Model file for the job. Use its own axes, mm. A direction names the side the tool comes from. Give positions to 0.01 mm unless a question says otherwise; leave off trailing zeros. Loops run counter-clockwise (first coordinate to the right, second up) from the corner with the lowest first, then second, coordinate; pieces in that order, holes last. Notation, with made-up numbers: (-34, 50) - (12, 50) arc R25 cw to (12, 80) - close; hole circle Ø6 at (12.25, 3). An arc over 180 degrees is marked (long way). Use a Markdown table: item, result.
from build123d import *

# Parameters (mm, degrees)
F0_W          = 12.7
F0_H          = 12.7
F1_DEPTH      = 16.51
F1_DEPTH_BACK = 16.51
F2_W          = 27.94
F2_H          = 6.35
F3_DEPTH      = 25.4
F5_DEPTH      = 27.94
F7_D          = 3.81
F8_R          = 3.81
F9_DEPTH      = 1.27


with BuildPart() as f1:
    # F0 (on Right) → F1 (new body, two sides)
    with BuildSketch(Plane.YZ) as f1_sk:
        Rectangle(F0_W, F0_H)
    extrude(amount=F1_DEPTH)
    extrude(f1_sk.sketch, amount=-F1_DEPTH_BACK)

    # F2 (on face) → F3 (cut)
    with BuildSketch(Plane.XZ.offset(6.35)):
        with Locations((0, -3.175)):
            Rectangle(F2_W, F2_H)
    extrude(amount=-F3_DEPTH, mode=Mode.SUBTRACT)

    # F4 (on face) → F5 (cut)
    with BuildSketch(Plane(origin=(13.97, 0, 0), x_dir=(0, -1, 0), z_dir=(-1, 0, 0))):
        with BuildLine():
            Line((-6.35, 0), (6.35, 0))
            ThreePointArc((6.35, 0), (0, 2.430635), (-6.35, 0))
        make_face()
    extrude(amount=F5_DEPTH, mode=Mode.SUBTRACT)

    # F7 (through all)
    with Locations(Plane.YZ.offset(16.51)):
        with Locations((0, -0.762)):
            Hole(F7_D / 2)

    # F8 (on face) → F9 (join)
    with BuildSketch(Plane.XY.offset(6.35)):
        with Locations((-10.16, 0)):
            Circle(F8_R)
        Circle(F8_R)
        with Locations((10.16, 0)):
            Circle(F8_R)
    extrude(amount=F9_DEPTH)


solid = f1.part
(1) Slice it at A-A, the plane z = -4.5. Write the cut outline in (x, y).
Computed:
| item | result |
|---|---|
| outline | (-16.51, -6.35) - (-13.97, -6.35) - (-13.97, 6.35) - (-16.51, 6.35) - close; (13.97, -6.35) - (16.51, -6.35) - (16.51, 6.35) - (13.97, 6.35) - close |
(2) Mould opens along Y. For faces 1 (the cylindrical face through (0.2, -0.1, 2.43)), 2 (the cylindrical face through (15.222, -1.817, -0.19)), 3 (the flat face through (0, 6.35, 3)), 4 (the cylindrical face through (6.354, 0.168, 6.976)) say: pulls with the +Y half, pulls with the -Y half, needs draft (parallel to the pull), parting line crosses it, or undercut.
Computed:
| item | result |
|---|---|
| face 1 | undercut |
| face 2 | undercut |
| face 3 | pulls with the +Y half |
| face 4 | parting line crosses it |
(3) Pin check, flat tips, straight feed: P1, Ø6, axis at y = 0, z = -0.762, coming from the +X side; P2, Ø3.5, axis at y = 0, z = -0.762, coming from the +X side; P3, Ø6, axis at x = 0, y = -2.5, coming from the -Z side. Stop position of each tip, or through.
Computed:
| item | result |
|---|---|
| P1 | x = 16.51 |
| P2 | through |
| P3 | z = 0.68 |
(4) Slice it at D-D, the plane y = -3. Write the cut outline in (x, z).
Computed:
| item | result |
|---|---|
| outline | (-16.51, -6.35) - (-13.97, -6.35) - (-13.97, 1.95) - (13.97, 1.95) - (13.97, -6.35) - (16.51, -6.35) - (16.51, 6.35) - (12.51, 6.35) - (12.51, 7.62) - (7.81, 7.62) - (7.81, 6.35) - (2.35, 6.35) - (2.35, 7.62) - (-2.35, 7.62) - (-2.35, 6.35) - (-7.81, 6.35) - (-7.81, 7.62) - (-12.51, 7.62) - (-12.51, 6.35) - (-16.51, 6.35) - close |
(5) Slice it at C-C, the plane x = 10.16. Write the cut outline in (y, z), plus the area to 3 significant figures.
Computed:
| item | result |
|---|---|
| outline | (-6.35, 0) arc R9.51 cw to (6.35, 0) - (6.35, 6.35) - (3.81, 6.35) - (3.81, 7.62) - (-3.81, 7.62) - (-3.81, 6.35) - (-6.35, 6.35) - close |
| area | 69.2 mm² |
(6) Slice it at B-B, the plane y = 0. Write the cut outline in (x, z), plus the area to 3 significant figures.
Computed:
| item | result |
|---|---|
| outline | (-16.51, -6.35) - (-13.97, -6.35) - (-13.97, -2.67) - (-16.51, -2.67) - close; (-16.51, 1.14) - (-13.97, 1.14) - (-13.97, 2.43) - (13.97, 2.43) - (13.97, 1.14) - (16.51, 1.14) - (16.51, 6.35) - (13.97, 6.35) - (13.97, 7.62) - (6.35, 7.62) - (6.35, 6.35) - (3.81, 6.35) - (3.81, 7.62) - (-3.81, 7.62) - (-3.81, 6.35) - (-6.35, 6.35) - (-6.35, 7.62) - (-13.97, 7.62) - (-13.97, 6.35) - (-16.51, 6.35) - close; (13.97, -6.35) - (16.51, -6.35) - (16.51, -2.67) - (13.97, -2.67) - close |
| area | 184 mm² |
(7) 3-axis set-ups, long thin cutter, end or side, ignore diameter. For faces 5 (the cylindrical face through (-6.526, 1.144, 6.976)), 6 (the flat face through (0, -6.35, 3)), 7 (the flat face through (13.97, 0, -3)): which of +Z, -Z, +X, -X, +Y, -Y reach the whole face in a straight line?
Computed:
| item | result |
|---|---|
| face 5 | +Z |
| face 6 | +Z, -Z, +X, -X, -Y |
| face 7 | -Z |
(8) Drill centre lines: probe 1 along Z at (x, y) = (15.05, 0); probe 2 along X at (y, z) = (-2.75, 0.75); probe 3 along X at (y, z) = (-1.5, 6.5). Where is each one in solid material? Low to high. Write a range as [from, to].
Computed:
| item | result |
|---|---|
| probe 1 | [-6.35, -2.67], [1.14, 6.35] |
| probe 2 | [-16.51, -13.97], [13.97, 16.51] |
| probe 3 | [-13.66, -6.66], [-3.5, 3.5], [6.66, 13.66] |
